Verification items for the finished model (mm, model axes). Give positions to 0.01 mm unless a question says otherwise; leave off trailing zeros. Write each loop counter-clockwise with the first axis right and the second up, starting at its lowest first coordinate (ties: lowest second). Pieces come first, ordered by that corner, then holes.
from build123d import *

# Parameters (mm, degrees)
SKETCH1_W           = 50
SKETCH1_H           = 700
BOSS_EXTRUDE1_DEPTH = 5
SKETCH6_R           = 3
CUT_EXTRUDE3_DEPTH  = 6
SKETCH11_W          = 10
SKETCH11_H          = 700
CUT_EXTRUDE4_DEPTH  = 3


with BuildPart() as part:
    # Sketch1 → Boss-Extrude1 (new body)
    with BuildSketch(Plane(origin=(0, 0, 0), x_dir=(1, 0, 0), z_dir=(0, 1, 0))):
        with Locations((25, 350)):
            Rectangle(SKETCH1_W, SKETCH1_H)
    extrude(amount=BOSS_EXTRUDE1_DEPTH)

    # Sketch6 → Cut-Extrude3 (cut, through all)
    with BuildSketch(Plane(origin=(0, 5, 0), x_dir=(1, 0, 0), z_dir=(0, 1, 0))):
        with Locations((43, 25)):
            Circle(SKETCH6_R)
        with Locations((7, 25)):
            Circle(SKETCH6_R)
        with Locations((43, 675)):
            Circle(SKETCH6_R)
        with Locations((7, 675)):
            Circle(SKETCH6_R)
    extrude(amount=-CUT_EXTRUDE3_DEPTH, mode=Mode.SUBTRACT)

    # Sketch11 → Cut-Extrude4 (cut)
    with BuildSketch(Plane.XZ):
        with Locations((7, -350)):
            Rectangle(SKETCH11_W, SKETCH11_H)
        with Locations((43, -350)):
            Rectangle(SKETCH11_W, SKETCH11_H)
    extrude(amount=-CUT_EXTRUDE4_DEPTH, mode=Mode.SUBTRACT)


solid = part.part
Item 1: Sectioned sample at B-B on z = -178.5. Record the cut outline in (x, y).
Answer key:
outline: (0, 0) - (2, 0) - (2, 3) - (12, 3) - (12, 0) - (38, 0) - (38, 3) - (48, 3) - (48, 0) - (50, 0) - (50, 5) - (0, 5) - close
Item 2: Depth check by flat-ended pin: pin 1 (5 mm diameter, centred on x = 22, z = -282, fed in from -Y); pin 2 (8 mm diameter, centred on x = 43, z = -675, fed in from -Y). Enter the tip coordinate at first touch or a pass-through.
Answer key:
pin 1: stops at y = 0
pin 2: stops at y = 3
Item 3: Scan lines: line 1 along X through (y, z) = (0.2, -357); line 2 along Z through (x, y) = (7, 4.15); line 3 along X through (y, z) = (4.5, -675). Record each from-to range of solid material in increasing order.
Answer key:
line 1: x = 0 to 2, 12 to 38, 48 to 50
line 2: z = -700 to -678, -672 to -28, -22 to 0
line 3: x = 0 to 4, 10 to 40, 46 to 50
Item 4: Sectioned sample at A-A on y = 1.5. Record the cut outline in (x, z).
Answer key:
outline: (0, -700) - (2, -700) - (2, 0) - (0, 0) - close; (12, -700) - (38, -700) - (38, 0) - (12, 0) - close; (48, -700) - (50, -700) - (50, 0) - (48, 0) - close
